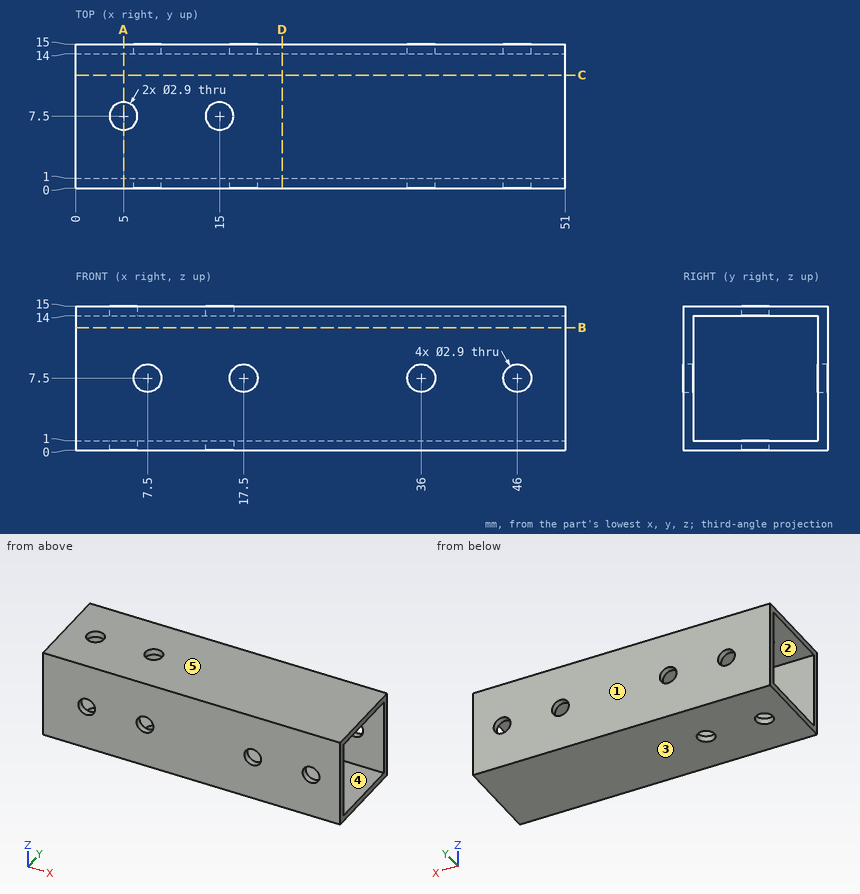
Check sheet for the drawn part. Datum: minimum x, y, z corner. Units: mm. A direction names the side the tool comes from. Give positions to 0.01 mm unless a question says otherwise; leave off trailing zeros. Write each loop counter-clockwise with the first axis right and the second up, starting at its lowest first coordinate (ties: lowest second). Pieces come first, ordered by that corner, then holes. Notation, with made-up numbers: (85.25, -31.5) - (139.25, -31.5) arc R29 cw to (139.25, 5.5) - close; hole circle Ø7 at (70.25, -21). An arc over 180 degrees is marked (long way). Put each result on its own line as item: value.
1. Set-up check for the marked faces 4 and 5: record each of +Z, -Z, +X, -X, +Y, -Y from which the full face is reachable in a straight line by a thin tool's end or side.
Ans:
face 4: +X, -X
face 5: +Z, +X, -X, +Y, -Y
2. Sectioned sample at A-A, the plane x = 5. Enter the section's corners in (y, z).
Ans:
outline: (0, 0) - (6.05, 0) - (6.05, 1) - (1, 1) - (1, 14) - (6.05, 14) - (6.05, 15) - (0, 15) - close; (8.95, 0) - (15, 0) - (15, 15) - (8.95, 15) - (8.95, 14) - (14, 14) - (14, 1) - (8.95, 1) - close
3. Sectioned sample at B-B, the plane z = 12.75. Enter the section's corners in (x, y), plus the area to 3 significant figures.
Ans:
outline: (0, 0) - (51, 0) - (51, 1) - (0, 1) - close; (0, 14) - (51, 14) - (51, 15) - (0, 15) - close
area: 102 mm²
4. Sectioned sample at D-D, the plane x = 21.5. Enter the section's corners in (y, z), plus the area to 3 significant figures.
Ans:
outline: (0, 0) - (15, 0) - (15, 15) - (0, 15) - close; hole (1, 1) - (14, 1) - (14, 14) - (1, 14) - close
area: 56.0 mm²
5. Thickness scan on line 1 (X direction, y = 14.45, z = 7.5); line 2 (Y direction, x = 26, z = 6.5). Record the ranges inside material, lowest first.
Ans:
line 1: x = 0 to 6.05, 8.95 to 16.05, 18.95 to 34.55, 37.45 to 44.55, 47.45 to 51
line 2: y = 0 to 1, 14 to 15
6. Go/stop test with a flat-tipped pin: pin 1 (1.7 mm diameter, centred on x = 46, z = 7.5, fed in from +Y). Record where the tip stops, or that it passes through.
Ans:
pin 1: passes through
7. Draft check along Z on the marked faces 1, 2 and 3. Enter one of: +Z half, -Z half, draft (parallel to the pull), parting line (faces both ways), or undercut.
Ans:
face 1: draft
face 2: undercut
face 3: -Z half
